Autodesk Fusion 360 part; units mm, degrees
sketch "Sketch1" plane through (0, 0, 0) normal (0, 0, 1) x (1, 0, 0)
  line L0 (0, 0) -> (35, 0)
  line L1 (35, 0) -> (35, 35)
  line L2 (35, 35) -> (0, 35)
  line L3 (0, 35) -> (0, 0)
  dimension "d1" = 35
  dimension "d2" = 35
extrude "Extrude1" add sketch "Sketch1" along normal blind 3
sketch "Sketch2" plane through (0, 0, 3) normal (0, 0, 1) x (-1, 0, 0)
  line L0 (0, -35) -> (0, 0)
  line L1 (0, 0) -> (-35, 0)
  line L2 (-35, 0) -> (-35, -35)
  line L3 (-35, -35) -> (0, -35)
  line L4 (-10, -35) -> (-35, -35)
  line L5 (-35, -35) -> (-35, -17.5)
  line L6 (-35, -17.5) -> (-10, -17.5)
  line L7 (-10, -17.5) -> (-10, -35)
  dimension "d5" = 25
  dimension "d6" = 17.5
extrude "Extrude2" cut sketch "Sketch2" against normal blind 3 contours L2 L3 L4 L5 L6 L7
sketch "Sketch6" plane through (0, 0, 3) normal (0, 0, 1) x (-1, 0, 0)
  line L0 (-35, -17.5) -> (-10, -17.5)
  line L1 (-10, -17.5) -> (-10, -35)
  line L2 (-10, -35) -> (0, -35)
  line L3 (0, -35) -> (0, 0)
  line L4 (0, 0) -> (-35, 0)
  line L5 (-35, 0) -> (-35, -17.5)
  line L6 (-10, -17.5) -> (-14, -17.5)
  line L7 (-14, -17.5) -> (-14, 0)
  line L8 (-14, 0) -> (-10, 0)
  line L9 (-10, 0) -> (-10, -17.5)
  dimension "d23" = 4
  dimension "d24" = 17.5
extrude "Extrude6" add sketch "Sketch6" along normal blind 6 contours L0 L4 L6 L7 L8 L9
extrude "Extrude7" cut 1 faces at (35, 5.8333, 1) along direction (-1, 0, 0) blind 5
sketch "Sketch7" plane through (0, 0, 3) normal (0, 0, 1) x (-1, 0, 0)
  line L0 (-30, 0) -> (-30, -17.5)
  line L1 (-30, -17.5) -> (-14, -17.5)
  line L2 (-14, -17.5) -> (-14, 0)
  line L3 (-14, 0) -> (-30, 0)
  line L4 (-30, -17.5) -> (-26, -17.5)
  line L5 (-26, -17.5) -> (-26, 0)
  line L6 (-26, 0) -> (-30, 0)
  line L7 (-30, 0) -> (-30, -17.5)
  dimension "d29" = 4
  dimension "d30" = 17.5
extrude "Extrude8" add sketch "Sketch7" along normal blind 6 contours L0 L1 L3 L4 L5 L6 L7
extrude "Extrude9" add 1 faces at (28.6667, 17.5, 4) along direction (0, 1, 0) blind 3.5
sketch "Sketch8" plane through (14, 0, 0) normal (1, 0, 0) x (0, 1, 0)
  line L0 (0, 3) -> (21, 3)
  line L1 (21, 3) -> (21, 9)
  line L2 (21, 9) -> (0, 9)
  line L3 (0, 9) -> (0, 3)
  line L4 (0, 7) -> (21, 7)
  line L5 (21, 7) -> (21, 5)
  line L6 (21, 5) -> (0, 5)
  line L7 (0, 5) -> (0, 7)
  dimension "d35" = 2
  dimension "d36" = 2
extrude "Extrude10" cut sketch "Sketch8" against normal blind 2 contours L1 L3 L4 L5 L6 L7
sketch "Sketch9" plane through (26, 0, 0) normal (-1, 0, 0) x (0, -1, 0)
  line L0 (-21, 3) -> (0, 3)
  line L1 (0, 3) -> (0, 9)
  line L2 (0, 9) -> (-21, 9)
  line L3 (-21, 9) -> (-21, 3)
  line L4 (-21, 7) -> (0, 7)
  line L5 (0, 7) -> (0, 5)
  line L6 (0, 5) -> (-21, 5)
  line L7 (-21, 5) -> (-21, 7)
  dimension "d39" = 2
  dimension "d40" = 2
extrude "Extrude11" cut sketch "Sketch9" against normal blind 2 contours L1 L3 L4 L5 L6 L7
sketch "Sketch10" plane through (0, 0, 5) normal (0, 0, 1) x (-1, 0, 0)
  line L0 (-26, -21) -> (-26, 0)
  line L1 (-26, 0) -> (-28, 0)
  line L2 (-28, 0) -> (-28, -21)
  line L3 (-28, -21) -> (-26, -21)
  line L4 (-26, 0) -> (-28, 0)
  line L5 (-28, 0) -> (-28, -2)
  line L6 (-28, -2) -> (-26, -2)
  line L7 (-26, -2) -> (-26, 0)
  dimension "d43" = 2
  dimension "d44" = 2
extrude "Extrude12" add sketch "Sketch10" along normal blind 2 contours L0 L1 L2 L4 L5 L6 L7
sketch "Sketch11" plane through (0, 0, 5) normal (0, 0, 1) x (-1, 0, 0)
  line L0 (-14, 0) -> (-14, -21)
  line L1 (-14, -21) -> (-12, -21)
  line L2 (-12, -21) -> (-12, 0)
  line L3 (-12, 0) -> (-14, 0)
  line L4 (-14, 0) -> (-12, 0)
  line L5 (-12, 0) -> (-12, -2)
  line L6 (-12, -2) -> (-14, -2)
  line L7 (-14, -2) -> (-14, 0)
  dimension "d47" = 2
  dimension "d48" = 2
extrude "Extrude13" add sketch "Sketch11" along normal blind 2 contours L0 L2 L3 L4 L5 L6 L7
sketch "Sketch14" plane through (0, 21, 0) normal (0, 1, 0) x (-1, 0, 0)
  line L0 (-26, 5) -> (-28, 5)
  line L1 (-28, 5) -> (-28, 7)
  line L2 (-28, 7) -> (-26, 7)
  line L3 (-26, 7) -> (-26, 9)
  line L4 (-26, 9) -> (-30, 9)
  line L5 (-30, 9) -> (-30, 0)
  line L6 (-30, 0) -> (-10, 0)
  line L7 (-10, 0) -> (-10, 3)
  line L8 (-10, 3) -> (-10, 9)
  line L9 (-10, 9) -> (-14, 9)
  line L10 (-14, 9) -> (-14, 7)
  line L11 (-14, 7) -> (-12, 7)
  line L12 (-12, 7) -> (-12, 5)
  line L13 (-12, 5) -> (-14, 5)
  line L14 (-14, 5) -> (-14, 3)
  line L15 (-14, 3) -> (-26, 3)
  line L16 (-26, 3) -> (-26, 5)
  line L17 (-10, 3) -> (-30, 3)
  line L18 (-30, 3) -> (-30, 0)
  line L19 (-30, 0) -> (-10, 0)
  line L20 (-10, 0) -> (-10, 3)
  dimension "d61" = 20
extrude "Extrude17" add sketch "Sketch14" along normal blind 10 contours L5 L6 L7 L15 L17 L18 L19 L20
extrude "Extrude18" cut 1 faces at (0, 23.3333, 1) along direction (1, 0, 0) blind 10
sketch "Sketch15" plane through (10, 0, 0) normal (-1, 0, 0) x (0, -1, 0)
  line L0 (0, 0) -> (0, 9)
  line L1 (0, 9) -> (-21, 9)
  line L2 (-21, 9) -> (-21, 3)
  line L3 (-21, 3) -> (-31, 3)
  line L4 (-31, 3) -> (-31, 0)
  line L5 (-31, 0) -> (0, 0)
  line L6 (-21, 3) -> (-31, 3)
  line L7 (-31, 3) -> (-31, 0)
  line L8 (-31, 0) -> (-21, 0)
  line L9 (-21, 0) -> (-21, 3)
extrude "Extrude19" add sketch "Sketch15" along normal blind 8 contours L3 L4 L5 L6 L7 L8 L9
sketch "Sketch16" plane through (30, 0, 0) normal (1, 0, 0) x (0, 1, 0)
  line L0 (21, 9) -> (0, 9)
  line L1 (0, 9) -> (0, 0)
  line L2 (0, 0) -> (31, 0)
  line L3 (31, 0) -> (31, 3)
  line L4 (31, 3) -> (21, 3)
  line L5 (21, 3) -> (21, 9)
  line L6 (21, 3) -> (31, 3)
  line L7 (31, 3) -> (31, 0)
  line L8 (31, 0) -> (21, 0)
  line L9 (21, 0) -> (21, 3)
  dimension "d68" = 10
extrude "Extrude20" add sketch "Sketch16" along normal blind 8 contours L2 L3 L4 L6 L7 L8 L9
sketch "Sketch17" plane through (0, 0, 0) normal (0, 0, -1) x (1, 0, 0)
  line L0 (10, 0) -> (10, -21)
  line L1 (10, -21) -> (2, -21)
  line L2 (2, -21) -> (2, -31)
  line L3 (2, -31) -> (38, -31)
  line L4 (38, -31) -> (38, -21)
  line L5 (38, -21) -> (30, -21)
  line L6 (30, -21) -> (30, 0)
  line L7 (30, 0) -> (10, 0)
  circle A0 centre (20, -26) radius 1.5
  dimension "d71" = 3
  dimension "d72" = 5
  dimension "d73" = 10
extrude "Extrude21" cut sketch "Sketch17" against normal blind 3 contours A0
sketch "Sketch18" plane through (0, 0, 0) normal (0, 0, -1) x (1, 0, 0)
  circle A0 centre (20, -26) radius 1.5
  line L0 (10, 0) -> (10, -21)
  line L1 (10, -21) -> (2, -21)
  line L2 (2, -21) -> (2, -31)
  line L3 (2, -31) -> (38, -31)
  line L4 (38, -31) -> (38, -21)
  line L5 (38, -21) -> (30, -21)
  line L6 (30, -21) -> (30, 0)
  line L7 (30, 0) -> (10, 0)
  circle A1 centre (6, -26) radius 1
  dimension "d76" = 2
  dimension "d77" = 14
extrude "Extrude22" cut sketch "Sketch18" against normal blind 3 contours A1
sketch "Sketch19" plane through (0, 0, 0) normal (0, 0, -1) x (1, 0, 0)
  circle A0 centre (6, -26) radius 1
  circle A1 centre (20, -26) radius 1.5
  line L0 (10, 0) -> (10, -21)
  line L1 (10, -21) -> (2, -21)
  line L2 (2, -21) -> (2, -31)
  line L3 (2, -31) -> (38, -31)
  line L4 (38, -31) -> (38, -21)
  line L5 (38, -21) -> (30, -21)
  line L6 (30, -21) -> (30, 0)
  line L7 (30, 0) -> (10, 0)
  circle A2 centre (34, -26) radius 1
  dimension "d80" = 2
  dimension "d81" = 14
  dimension "d82" = 5
extrude "Extrude23" cut sketch "Sketch19" against normal blind 3 contours A2
fillet "Fillet1" radius 5 1 edges at (38, 21, 1.5)
fillet "Fillet2" radius 5 1 edges at (38, 31, 1.5)
fillet "Fillet3" radius 5 1 edges at (2, 31, 1.5)
fillet "Fillet4" radius 5 1 edges at (2, 21, 1.5)
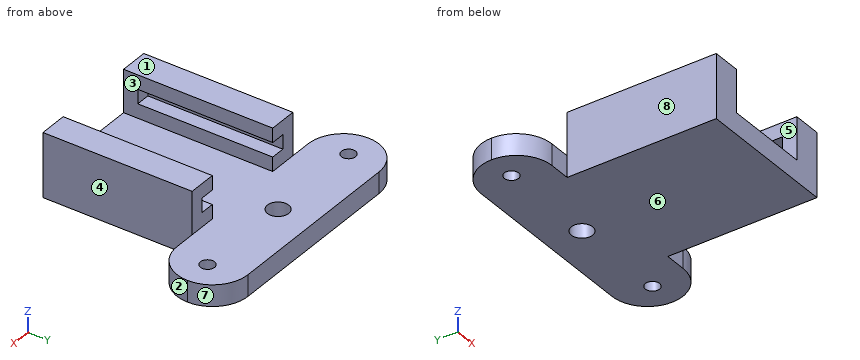
The model under review builds one solid part; all positions refer to its coordinate system, in mm. Face numbers are marked on the shaded views. A direction names the side the tool comes from. Give positions to 0.01 mm unless a question says otherwise; leave off trailing zeros. Order: outer loops, then holes, each group sorted by start corner. A loop starts at its lowest first (then second) coordinate and runs counter-clockwise, first axis right, second up. Notation, with made-up numbers: (14.25, -39) - (39.25, -39) arc R15 cw to (39.25, -17) - close; hole circle Ø3 at (29.5, 26). An arc over 180 degrees is marked (long way). Use CSV: the item, a comma, the result in double quotes. Start each with the question number.
Q1. We need section B-B, the plane x = 20. Write out the cut boundary in (y, z).
Q2. Clearance check with flat-ended pins moving along their axes: pin 1 Ø2.5 at (x, y) = (6, 26) entering from +Z; pin 2 Ø4.5 at (y, z) = (12, 5.5) entering from +X; pin 3 Ø2 at (x, z) = (28.5, 6) entering from +Y. State where each tip first meets the part, or that it passes through.
Q3. Tool access review of the marked faces 4, 5, 6, 7 and 8: name each direction out of +Z, -Z, +X, -X, +Y, -Y from which nothing blocks a thin tool from reaching the whole face with its end or side.
Q4. The part is to be moulded in two halves that separate along X. For the marked faces 1, 2 and 3, say which applies: +X half, -X half, draft (parallel to the pull), parting line (faces both ways), or undercut.
Q5. To check wall thickness, follow line 1 along X through (y, z) = (26, 1.5); line 2 along Z through (x, y) = (12.5, 8); line 3 along Y through (x, z) = (20, 2.05). State the ranges of each line that lie inside material, in increasing order. Write a range as [from, to].
Q6. We need section C-C, the plane y = 7. Write out the cut boundary in (x, z), and give its area (3 significant figures).
Q7. We need section D-D, the plane x = 12.5. Write out the cut boundary in (y, z), and give its area (3 significant figures).
Q8. We need section A-A, the plane z = 6. Write out the cut boundary in (x, y), and give its area (3 significant figures).
Outcome:
1,outline,"(0, 0) - (24.5, 0) - (24.5, 3) - (0, 3) - close; (27.5, 0) - (31, 0) - (31, 3) - (27.5, 3) - close"
2,pin 1,"stops at z = 3"
2,pin 2,"stops at x = 30"
2,pin 3,"stops at y = 21"
3,face 4,"+Z, -Z, +X, -Y"
3,face 5,"+Z, +Y, -Y"
3,face 6,"-Z, +X, -X, +Y, -Y"
3,face 7,"+Z, -Z, +X, +Y"
3,face 8,"+Z, -Z, -X, -Y"
4,face 1,"draft"
4,face 2,"+X half"
4,face 3,"undercut"
5,line 1,"x = [2, 5], [7, 18.5], [21.5, 33], [35, 38]"
5,line 2,"z = [0, 5], [7, 9]"
5,line 3,"y = [0, 24.5], [27.5, 31]"
6,outline,"(10, 0) - (30, 0) - (30, 9) - (26, 9) - (26, 7) - (28, 7) - (28, 5) - (26, 5) - (26, 3) - (14, 3) - (14, 5) - (12, 5) - (12, 7) - (14, 7) - (14, 9) - (10, 9) - close"
6,area,"100 mm^2"
7,outline,"(0, 0) - (31, 0) - (31, 3) - (21, 3) - (21, 5) - (2, 5) - (2, 7) - (21, 7) - (21, 9) - (0, 9) - close"
7,area,"181 mm^2"
8,outline,"(10, 0) - (14, 0) - (14, 2) - (12, 2) - (12, 21) - (10, 21) - close; (26, 0) - (30, 0) - (30, 21) - (28, 21) - (28, 2) - (26, 2) - close"
8,area,"92.0 mm^2"
